Geometry: final body of the model. Coordinates: model frame, mm. Coordinates: 2 decimals unless noted, no trailing zeros. Order: outer loops, then holes, each group sorted by start corner. A loop starts at its lowest first (then second) coordinate and runs counter-clockwise, first axis right, second up. Notation, with made-up numbers: (31, -15.75) - (41, -15.75) arc R34 ccw to (41, 20.25) - close; hole circle Ø1 at (34.5, 76). An arc over 180 degrees is marked (long way). Use a Markdown table: item, result. Add a question column.
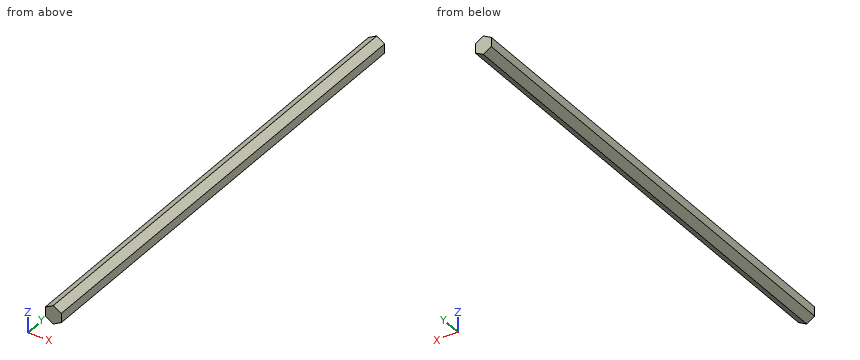
Autodesk Inventor part; units mm, degrees
ref_plane "YZ Plane" through (0, 0, 0) normal (1, 0, 0) x (0, 1, 0)
ref_plane "XZ Plane" through (0, 0, 0) normal (0, 1, 0) x (-1, 0, 0)
ref_plane "XY Plane" through (0, 0, 0) normal (0, 0, 1) x (1, 0, 0)
sketch "Sketch1" plane through (0, 0, 0) normal (0, 1, 0) x (-1, 0, 0)
  line L0 (0, -7.3323) -> (-6.35, -3.6662)
  line L1 (-6.35, -3.6662) -> (-6.35, 3.6662)
  line L2 (-6.35, 3.6662) -> (0, 7.3323)
  line L3 (0, 7.3323) -> (6.35, 3.6662)
  line L4 (6.35, 3.6662) -> (6.35, -3.6662)
  line L5 (6.35, -3.6662) -> (0, -7.3323)
  point P0 (0, 0)
  point P1 (0, 0)
  dimension "d0" = 12.7
extrude "Extrusion1" add sketch "Sketch1" along normal blind 368.3
1) Section A-A (y = 34.5). Return loops of the section in (x, z), then the cut area to 3 significant figures.
2) Ray query, line 1 along X through (y, z) = (174, -5.25); line 2 along Z through (x, y) = (0.25, 80); line 3 along Z through (x, y) = (2, 32). Return the intervals inside material, ascending.
3) Section B-B (x = -3). Return loops of the section in (y, z).
4) Pin query (flat end, axial travel): pin 1 (1 mm diameter, centred on x = -1, y = 149.5, fed in from +Z); pin 2 (4 mm diameter, centred on x = -5, y = 61.5, fed in from +Z); pin 3 (1.5 mm diameter, centred on x = -3.5, y = 106, fed in from +Z). Return the tip coordinate at first contact, or that it passes through.
Values follow:
| question | item | result |
|---|---|---|
| 1 | outline | (-6.35, -3.67) - (0, -7.33) - (6.35, -3.67) - (6.35, 3.67) - (0, 7.33) - (-6.35, 3.67) - close |
| 1 | area | 140 mm² |
| 2 | line 1 | x = -3.61 to 3.61 |
| 2 | line 2 | z = -7.19 to 7.19 |
| 2 | line 3 | z = -6.18 to 6.18 |
| 3 | outline | (0, -5.6) - (368.3, -5.6) - (368.3, 5.6) - (0, 5.6) - close |
| 4 | pin 1 | stops at z = 7.04 |
| 4 | pin 2 | stops at z = 5.6 |
| 4 | pin 3 | stops at z = 5.74 |
